Here's how the part is built. I have some questions about the finished solid (model axes, mm). Coordinates: 2 decimals unless noted, no trailing zeros. Write each loop counter-clockwise with the first axis right and the second up, starting at its lowest first coordinate (ties: lowest second). Pieces come first, ordered by that corner, then holes. Notation, with made-up numbers: (85.5, 33.25) - (95.5, 33.25) arc R21 ccw to (95.5, 72.25) - close; hole circle Ø10 at (-29, 79). An arc over 180 degrees is marked (long way). Answer in a Markdown table with one row per item. Add a question column.
Item 1: If I drill on probe 1 along Y at (x, z) = (128, 13); probe 2 along X at (y, z) = (-559, 14.5); probe 3 along X at (y, z) = (-146, 17), over which ranges is the centre line in solid material (lowest first)? Write a range as from..to.
Item 2: I'm going to push flat-ended pins straight in: pin 1 (8 mm diameter, centred on y = -718.5, z = 33.5, fed in from -X); pin 2 (10 mm diameter, centred on y = -295, z = 29, fed in from +X); pin 3 (12 mm diameter, centred on y = -439, z = 15.5, fed in from -X). Where does each tip first touch, or does it pass through?
Item 3: Imagine slicing it at C-C (z = 34). Please give me the cut outline in (x, y), plus the area to 3 significant figures.
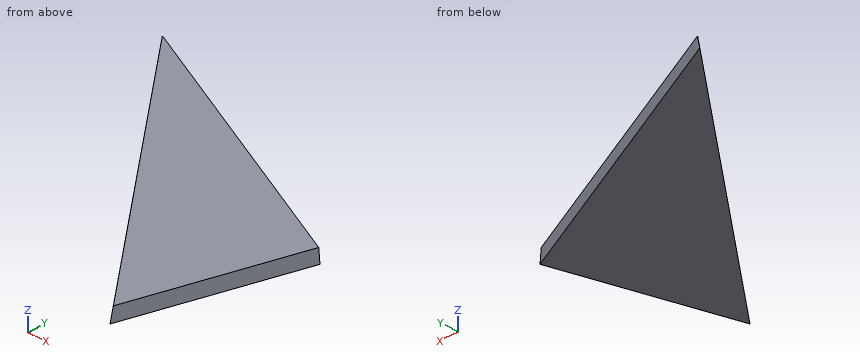
from build123d import *

# Parameters (mm, degrees)
EXTRUDE_1_DEPTH    = 60
CHAMFER3_SIZE2     = 11.912970931
CHAMFER3_SIZE      = 60
CHAMFER4_SIZE2     = 11.912970931
CHAMFER4_SIZE      = 60
CHAMFER5_SIZE2     = 9.519169095
CHAMFER5_SIZE      = 60
CUT_EXTRUDE2_DEPTH = 2201.39802191


with BuildPart() as part:
    # Эскиз1 → Бобышка-Вытянуть1 (new body)
    with BuildSketch(Plane.XY):
        Polygon((-849.589927609, 515.838957491), (787.506047005, 606.405063543), (281.615569427, -953.197537878), align=None)
    extrude(amount=EXTRUDE_1_DEPTH)

    # Chamfer3
    chamfer3_edges = [part.edges().sort_by_distance(p)[0] for p in [
        (-31.041940302, 561.122010517, 60),
    ]]
    chamfer3_side = [part.faces().sort_by_distance(p)[0] for p in [
        (-31.041940302, 561.122010517, 59.761740581),
    ]]
    chamfer(chamfer3_edges, length=CHAMFER3_SIZE - 0.0001, length2=CHAMFER3_SIZE2 - 0.0001, reference=chamfer3_side[0])  # a hair under: the kernel refuses the full size

    # Chamfer4
    chamfer4_edges = [part.edges().sort_by_distance(p)[0] for p in [
        (532.590398399, -179.470785737, 60),
    ]]
    chamfer4_side = [part.faces().sort_by_distance(p)[0] for p in [
        (532.590398399, -179.470785737, 59.761740581),
    ]]
    chamfer(chamfer4_edges, length=CHAMFER4_SIZE - 0.0001, length2=CHAMFER4_SIZE2 - 0.0001, reference=chamfer4_side[0])  # a hair under: the kernel refuses the full size

    # Chamfer5
    chamfer5_edges = [part.edges().sort_by_distance(p)[0] for p in [
        (-283.987179091, -218.679290193, 60),
    ]]
    chamfer5_side = [part.faces().sort_by_distance(p)[0] for p in [
        (-283.987179091, -218.679290193, 59.809616618),
    ]]
    chamfer(chamfer5_edges, length=CHAMFER5_SIZE - 0.0001, length2=CHAMFER5_SIZE2 - 0.0001, reference=chamfer5_side[0])  # a hair under: the kernel refuses the full size

    # 3DSketch1 → Cut-Extrude2 (cut, through all)
    with BuildSketch(Plane(origin=(-849.589927609, 515.838957491, 0), x_dir=(0.9984732860919079, 0.05523673560980175, 0), z_dir=(0, 0, -1))):
        Polygon((0, 0), (1343.966431425, 764.63889794), (1639.599173476, 0), align=None)
    extrude(amount=-CUT_EXTRUDE2_DEPTH, mode=Mode.SUBTRACT)


solid = part.part
Here are the results:
| question | item | result |
|---|---|---|
| 1 | probe 1 | y = -750.32..29.05 |
| 1 | probe 2 | x = -19.03..406.46 |
| 1 | probe 3 | x = -336.55..479.54 |
| 2 | pin 1 | stops at x = 104.42 |
| 2 | pin 2 | stops at x = 490.99 |
| 2 | pin 3 | stops at x = -116 |
| 3 | outline | (-838.07, 509.72) - (278.64, -940.49) - (528.45, -170.35) - (-837.37, 509.75) - close |
| 3 | area | 611,000 mm2 |
